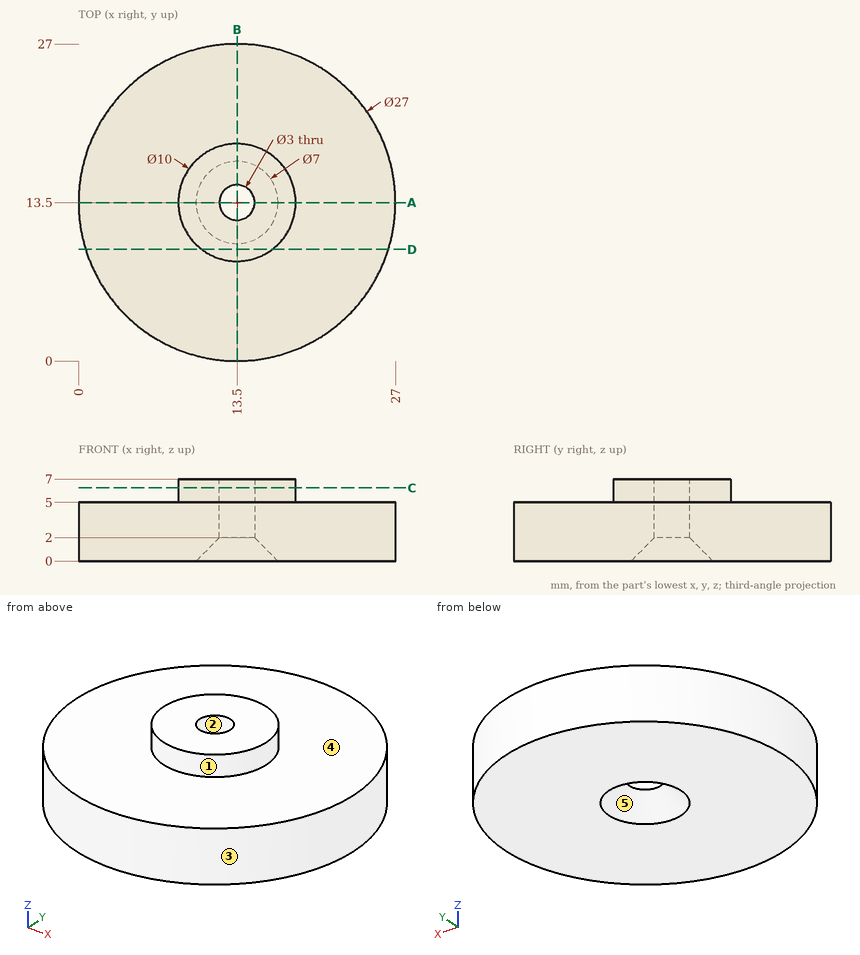
Could you check a few things on this drawing? It's one solid part, dimensions in mm from its lowest x, y, z. A direction names the side the tool comes from. Coordinates: 2 decimals unless noted, no trailing zeros. Order: outer loops, then holes, each group sorted by start corner. A loop starts at its lowest first (then second) coordinate and runs counter-clockwise, first axis right, second up. Notation, with made-up numbers: M -1.5,25 L 56.5,25 A7 ccw 56.5,33 Z; hole C 62.5,48 d10. An arc over 180 degrees is marked long. Use a Markdown table: item, result. Add a question column.
Q1. I'm going to push flat-ended pins straight in: pin 1 (1 mm diameter, centred on x = 3.5, z = 2, fed in from -Y); pin 2 (2 mm diameter, centred on x = 12.5, y = 4, fed in from +Z). Where does each tip first touch, or does it pass through?
Q2. I want a section at D-D on y = 9.5. List the corners of the cut face in (x, z) for me.
Q3. Which directions (+Z, -Z, +X, -X, +Y, -Y) give clear straight access to the entire face, cutting with the end or side of a thin tool? Please do the marked faces 1 and 2.
Q4. If I drill on L1, parallel to Y at x = 13.5, z = 3.6; L2, parallel to Z at x = 22.25, y = 11; L3, parallel to X at y = 13, z = 5.75, over which ranges is the centre line in solid material (lowest first)?
Q5. I want a section at A-A on y = 13.5. List the corners of the cut face in (x, z) for me, then the cut area to 3 significant figures.
Q6. We'd pull the mould along X, two halves only. Please class the marked faces 3, 4 and 5: pulls with the +X half, pulls with the -X half, needs draft (parallel to the pull), parting line crosses it, or undercut.
Q7. I want a section at C-C on z = 6.25. List the corners of the cut face in (x, y) for me.
Checked values:
| question | item | result |
|---|---|---|
| 1 | pin 1 | y = 3.91 |
| 1 | pin 2 | z = 5 |
| 2 | outline | M 0.61,0 L 26.39,0 L 26.39,5 L 16.5,5 L 16.5,7 L 10.5,7 L 10.5,5 L 0.61,5 Z |
| 3 | face 1 | +Z |
| 3 | face 2 | +Z, -Z |
| 4 | L1 | 0 to 12, 15 to 27 |
| 4 | L2 | 0 to 5 |
| 4 | L3 | 8.53 to 12.09, 14.91 to 18.47 |
| 5 | outline | M 0,0 L 10,0 L 12,2 L 12,7 L 8.5,7 L 8.5,5 L 0,5 Z; M 15,2 L 17,0 L 27,0 L 27,5 L 18.5,5 L 18.5,7 L 15,7 Z |
| 5 | area | 130 mm² |
| 6 | face 3 | parting line crosses it |
| 6 | face 4 | needs draft |
| 6 | face 5 | undercut |
| 7 | outline | C 13.5,13.5 d10; hole C 13.5,13.5 d3 |
